Input: part model. Units: mm. Frame: model coordinates. Coordinates: 2 decimals unless noted, no trailing zeros. Loops run counter-clockwise (first coordinate to the right, second up) from the corner with the lowest first, then second, coordinate; pieces in that order, holes last. Notation, with made-up numbers: (-19.5, 87) -> (9.5, 87) arc R15 ccw to (9.5, 100) -> close; hole circle Ø1 at (38, 59). An arc over 180 degrees is marked (long way). Put each result on its own line as item: value. Start each with the question number.
1) Material intervals for L1, parallel to Z at x = 16, y = 0.25; L2, parallel to X at y = 0.6, z = 6; L3, parallel to Z at x = 52, y = 1.4, sorted ascending.
2) Cut plane B-B (z = 39.5). Return the cut outline in (x, y).
3) Cut plane D-D (x = 49). Return the cut outline in (y, z).
4) Cut plane C-C (y = 1.4). Return the cut outline in (x, z).
5) Cut plane A-A (x = 16). Return the cut outline in (y, z).
6) Contact query for flat-ended pins moving along their axis: P1, Ø12, axis at x = 6, z = 30, coming from the -Y side; P2, Ø5, axis at x = 23.5, z = 24, coming from the +Y side; P3, Ø4, axis at x = 11.5, z = 26, coming from the +Y side; P4, Ø7.5, axis at x = 16, z = 6, coming from the +Y side. Output: stop coordinate, or through.
from build123d import *

# Parameters (mm, degrees)
BOSS_EXTRUDE1_DEPTH = 43
CUT_EXTRUDE1_REACH  = 4
SKETCH2_R           = 3.35


with BuildPart() as part:
    # Sketch1 → Boss-Extrude1 (new body)
    with BuildSketch(Plane.XY):
        Polygon((0, 0), (56.71, 0), (56.71, 2), align=None)
    extrude(amount=BOSS_EXTRUDE1_DEPTH)

    # Cut-Extrude1: up to this face of the body (flat: up to its plane)
    cut_extrude1_end = Plane(part.part.faces().sort_by_distance((28.355, 1, 21.5))[0])
    # Sketch2 → Cut-Extrude1 (cut, up to the picked face)
    with BuildSketch(Plane.XZ, mode=Mode.PRIVATE) as cut_extrude1_sk1:
        with Locations((49, 6)):
            Circle(SKETCH2_R)
    cut_extrude1_tool1 = split(extrude(cut_extrude1_sk1.sketch, amount=-CUT_EXTRUDE1_REACH, mode=Mode.PRIVATE), bisect_by=cut_extrude1_end, keep=Keep.BOTH, mode=Mode.PRIVATE)
    add(cut_extrude1_tool1.solids().sort_by_distance((49, 0, 6))[0], mode=Mode.SUBTRACT)
    # Sketch2 → Cut-Extrude1 (cut, up to the picked face)
    with BuildSketch(Plane.XZ, mode=Mode.PRIVATE) as cut_extrude1_sk2:
        with Locations((49, 37)):
            Circle(SKETCH2_R)
    cut_extrude1_tool2 = split(extrude(cut_extrude1_sk2.sketch, amount=-CUT_EXTRUDE1_REACH, mode=Mode.PRIVATE), bisect_by=cut_extrude1_end, keep=Keep.BOTH, mode=Mode.PRIVATE)
    add(cut_extrude1_tool2.solids().sort_by_distance((49, 0, 37))[0], mode=Mode.SUBTRACT)
    # Sketch2 → Cut-Extrude1 (cut, up to the picked face)
    with BuildSketch(Plane.XZ, mode=Mode.PRIVATE) as cut_extrude1_sk3:
        with Locations((16, 37)):
            Circle(SKETCH2_R)
    cut_extrude1_tool3 = split(extrude(cut_extrude1_sk3.sketch, amount=-CUT_EXTRUDE1_REACH, mode=Mode.PRIVATE), bisect_by=cut_extrude1_end, keep=Keep.BOTH, mode=Mode.PRIVATE)
    add(cut_extrude1_tool3.solids().sort_by_distance((16, 0, 37))[0], mode=Mode.SUBTRACT)
    # Sketch2 → Cut-Extrude1 (cut, up to the picked face)
    with BuildSketch(Plane.XZ, mode=Mode.PRIVATE) as cut_extrude1_sk4:
        with Locations((16, 6)):
            Circle(SKETCH2_R)
    cut_extrude1_tool4 = split(extrude(cut_extrude1_sk4.sketch, amount=-CUT_EXTRUDE1_REACH, mode=Mode.PRIVATE), bisect_by=cut_extrude1_end, keep=Keep.BOTH, mode=Mode.PRIVATE)
    add(cut_extrude1_tool4.solids().sort_by_distance((16, 0, 6))[0], mode=Mode.SUBTRACT)


solid = part.part
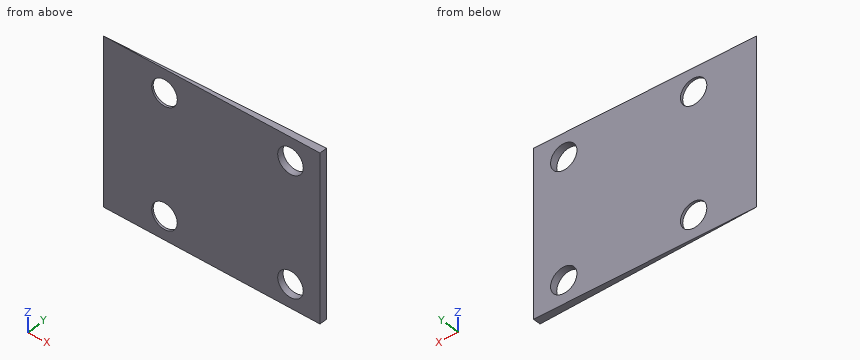
Results found:
1. L1: z = 0 to 2.65, 9.35 to 33.65, 40.35 to 43
1. L2: x = 19.35 to 45.65, 52.35 to 56.71
1. L3: z = 0 to 4.51, 7.49 to 35.51, 38.49 to 43
2. outline: (0, 0) -> (13.77, 0) -> (13.77, 0.49) -> close; (18.23, 0) -> (46.77, 0) -> (46.77, 1.65) -> (18.23, 0.64) -> close; (51.23, 0) -> (56.71, 0) -> (56.71, 2) -> (51.23, 1.81) -> close
3. outline: (0, 0) -> (1.73, 0) -> (1.73, 2.65) -> (0, 2.65) -> close; (0, 9.35) -> (1.73, 9.35) -> (1.73, 33.65) -> (0, 33.65) -> close; (0, 40.35) -> (1.73, 40.35) -> (1.73, 43) -> (0, 43) -> close
4. outline: (39.7, 0) -> (56.71, 0) -> (56.71, 43) -> (39.7, 43) -> close; hole circle Ø6.7 at (49, 6); hole circle Ø6.7 at (49, 37)
5. outline: (0, 0) -> (0.56, 0) -> (0.56, 2.65) -> (0, 2.65) -> close; (0, 9.35) -> (0.56, 9.35) -> (0.56, 33.65) -> (0, 33.65) -> close; (0, 40.35) -> (0.56, 40.35) -> (0.56, 43) -> (0, 43) -> close
6. P1: stops at y = 0
6. P2: stops at y = 0.92
6. P3: stops at y = 0.48
6. P4: stops at y = 0.7
